from build123d import *

# Parameters (mm, degrees)
SKETCH_1_R      = 0.95
EXTRUDE_1_DEPTH = 3
EXTRUDE_2_DEPTH = 5.2


with BuildPart() as part:
    # 草图1 → 凸台-拉伸1 (new body)
    with BuildSketch(Plane.XY):
        with BuildLine():
            Line((5.942462138, -8.684131796), (15.917990129, -4.533184225))
            ThreePointArc((15.917990129, -4.533184225), (18.153297697, -2.694164403), (18.992427879, 0.076116155))
            Line((18.992427879, 0.076116155), (18.992427879, 4.276025841))
            Line((18.992427879, 4.276025841), (0, 4.049500215))
            Line((0, 4.049500215), (-18.992427879, 4.276025841))
            Line((-18.992427879, 4.276025841), (-18.992427879, 0.076116155))
            ThreePointArc((-18.992427879, 0.076116155), (-18.153297697, -2.694164403), (-15.917990129, -4.533184225))
            Line((-15.917990129, -4.533184225), (-5.942462138, -8.684131796))
            ThreePointArc((-5.942462138, -8.684131796), (0, -10.002483291), (5.942462138, -8.684131796))
        make_face()
        with Locations((-14, 0.076116155)):
            Circle(SKETCH_1_R, mode=Mode.SUBTRACT)
        with Locations((14, 0.076116155)):
            Circle(SKETCH_1_R, mode=Mode.SUBTRACT)
        with Locations((0, -6.834517122)):
            Circle(SKETCH_1_R, mode=Mode.SUBTRACT)
    extrude(amount=EXTRUDE_1_DEPTH)

    # 草图2 → 凸台-拉伸2 (add)
    with BuildSketch(Plane(origin=(0, 0, 0), x_dir=(-1, 0, 0), z_dir=(0, 0, -1))):
        with BuildLine():
            ThreePointArc((-18.992427879, 0.076116155), (-18.153297697, -2.694164403), (-15.917990129, -4.533184225))
            Line((-15.917990129, -4.533184225), (-15.690391283, -3.98622028))
            ThreePointArc((-15.690391283, -3.98622028), (-17.66044544, -2.36542827), (-18.4, 0.076116155))
            Line((-18.4, 0.076116155), (-18.992427879, 0.076116155))
        make_face()
        Polygon((3.999715516, 4.097205441), (0, 4.049500215), (0, 0.076116155), (3.999715516, 0), align=None)
    extrude(amount=EXTRUDE_2_DEPTH)


solid = part.part
Could you check a few things on this model? Use its own coordinates, in mm. A direction names the side the tool comes from. Round coordinates to 2 decimals unless told otherwise and drop trailing zeros. Loops run counter-clockwise (first coordinate to the right, second up) from the corner with the lowest first, then second, coordinate; pieces in that order, holes last. Notation, with made-up numbers: (-11, -38) -> (19, -38) arc R13 cw to (19, -32) -> close; hole circle Ø8 at (73.5, 73). An arc over 180 degrees is marked (long way). Use CSV: the item, a comma, the result in double quotes.
(1) Will these pins go through, and if not, where does the flat tip stop? pin 1 Ø1.2 at (y, z) = (2, -1.5) entering from -X; pin 2 Ø4 at (x, z) = (8.5, -0.5) entering from +Y; pin 3 Ø3 at (x, y) = (0, -6.83) entering from -Z.
Return value:
pin 1,"stops at x = -4"
pin 2,"stops at y = 4.17"
pin 3,"stops at z = 0"
(2) Suppose I cut it at A-A on z = -2.5. Write out the boundary of the cut face in (x, y).
Return value:
outline,"(-4, 0) -> (0, 0.08) -> (0, 4.05) -> (-4, 4.1) -> close; (15.69, -3.99) -> (15.92, -4.53) arc R4.99 ccw to (18.99, 0.08) -> (18.4, 0.08) arc R4.4 cw to start"
(3) If I drill on probe 1 along Y at (x, z) = (0, 2.45); probe 2 along Z at (x, y) = (-11, 0.25); probe 3 along Y at (x, z) = (14, 1.4), over which ranges is the centre line in solid material (lowest first)? Write a range as [from, to].
Return value:
probe 1,"y = [-10, -7.78], [-5.88, 4.05]"
probe 2,"z = [0, 3]"
probe 3,"y = [-5.33, -0.87], [1.03, 4.22]"
(4) Suppose I cut it at D-D on x = -3. Write out the boundary of the cut face in (y, z).
Return value:
outline,"(-9.68, 0) -> (0.02, 0) -> (0.02, -5.2) -> (4.09, -5.2) -> (4.09, 3) -> (-9.68, 3) -> close"
(5) Suppose I cut it at C-C on z = 2.5. Write out the boundary of the cut face in (x, y), plus the area to 3 significant figures.
Return value:
outline,"(-18.99, 0.08) arc R4.99 ccw to (-15.92, -4.53) -> (-5.94, -8.68) arc R14.05 ccw to (5.94, -8.68) -> (15.92, -4.53) arc R4.99 ccw to (18.99, 0.08) -> (18.99, 4.28) -> (0, 4.05) -> (-18.99, 4.28) -> close; hole circle Ø1.9 at (-14, 0.08); hole circle Ø1.9 at (0, -6.83); hole circle Ø1.9 at (14, 0.08)"
area,"415 mm²"
(6) For faces 1 (the flat face through (-4, 2, -3)), 2 (the flat face through (0, -1, 3)), which set-ups out of +Z, -Z, +X, -X, +Y, -Y let a thin tool reach every point of the face, with its end or its side?
Return value:
face 1,"-Z, -X, +Y, -Y"
face 2,"+Z, +X, -X, +Y, -Y"
(7) If we mould it in two halves opening along Y, with no side actions, what happens to faces 3 (the flat face through (0, 2, -3)), 4 (the cylindrical face through (14.906, 0.361, 1.479)), 5 (the cylindrical face through (-13.094, 0.361, 1.479)), 6 (the cylindrical face through (-0.086, -10.002, 1.479))? For each: +Y half, -Y half, draft (parallel to the pull), parting line (faces both ways), or undercut.
Return value:
face 3,"draft"
face 4,"undercut"
face 5,"undercut"
face 6,"-Y half"
(8) Suppose I cut it at B-B on x = -13.5. Write out the boundary of the cut face in (y, z), plus the area to 3 significant figures.
Return value:
outline,"(-5.54, 0) -> (-0.73, 0) -> (-0.73, 3) -> (-5.54, 3) -> close; (0.88, 0) -> (4.21, 0) -> (4.21, 3) -> (0.88, 3) -> close"
area,"24.4 mm²"
